from build123d import *

# Parameters (mm, degrees)
SALIENTE_EXTRUIR1_DEPTH = 12


with BuildPart() as part:
    # Croquis1 → Saliente-Extruir1 (new body)
    with BuildSketch(Plane(origin=(0, 0, 0), x_dir=(1, 0, 0), z_dir=(0, 1, 0))):
        with BuildLine():
            Line((-237.438208893, 168.650156508), (-237.438208893, -9.106373442))
            Line((-237.438208893, -9.106373442), (-2.121320344, -9.106373442))
            ThreePointArc((-2.121320344, -9.106373442), (0, -9.106373442), (0, -11.227693785))
            Line((0, -11.227693785), (0, -21.106373442))
            Line((0, -21.106373442), (31, -21.106373442))
            Line((31, -21.106373442), (62, -21.106373442))
            Line((62, -21.106373442), (62, -11.227693785))
            ThreePointArc((62, -11.227693785), (62, -9.106373442), (64.121320344, -9.106373442))
            Line((64.121320344, -9.106373442), (299.438208893, -9.106373442))
            Line((299.438208893, -9.106373442), (299.438208893, 168.650156508))
            add(Edge.make_bspline(
                [(299.438208893, 168.650156508), (165.219104447, 12), (31, 12)],
                knots=[0, 0, 0, 1, 1, 1], degree=2))
            add(Edge.make_bspline(
                [(31, 12), (-103.219104447, 12), (-237.438208893, 168.650156508)],
                knots=[0, 0, 0, 1, 1, 1], degree=2))
        make_face()
    extrude(amount=SALIENTE_EXTRUIR1_DEPTH)


solid = part.part
CAD build for the part. Positions are in the model's coordinates, mm. A direction names the side the tool comes from. Give positions to 0.01 mm unless a question says otherwise; leave off trailing zeros. Put each result on its own line as item: value. Start each with the question number.
(1) Probe L1, parallel to X at y = 0.5, z = -113.5; L2, parallel to X at y = 8, z = -153; L3, parallel to Z at x = -91, y = 10. List the from-to ranges inside material, lowest first.
(2) Which spindle directions (+Z, -Z, +X, -X, +Y, -Y) get a long thin tool onto all of the face, cutting with end or side? Do faces 1 (the face through (62, 6, 16)), 2 (the face through (-121, 6, 9.106)), 3 (the face through (10, 0, -1)). Say none if no direction does.
(3) Flat gauge pins, fed straight in: pin 1 Ø1 at (x, y) = (164.5, 5.5) entering from -Z; pin 2 Ø5 at (x, y) = (-182.5, 10) entering from +Z; pin 3 Ø3 at (y, z) = (4.5, 15.5) entering from -X. Where does each tip first touch, or does it go through?
Response values:
1. L1: x = -237.44 to -185.08, 247.08 to 299.44
1. L2: x = -237.44 to -223.68, 285.68 to 299.44
1. L3: z = -44.36 to 9.11
2. face 1: +Z, +X, +Y, -Y
2. face 2: +Z, -X, +Y, -Y
2. face 3: +Z, -Z, +X, -X, -Y
3. pin 1: stops at z = -51.03
3. pin 2: stops at z = 9.11
3. pin 3: stops at x = 0
